```python
from build123d import *

# Parameters (mm, degrees)
SKETCH1_W           = 100
SKETCH1_H           = 20
BOSS_EXTRUDE1_DEPTH = 3
FILLET1_R           = 0.5
SKETCH2_R           = 1.5
CUT_EXTRUDE1_DEPTH  = 4


with BuildPart() as part:
    # Sketch1 → Boss-Extrude1 (new body)
    with BuildSketch(Plane(origin=(0, 0, 0), x_dir=(1, 0, 0), z_dir=(0, 1, 0))):
        Rectangle(SKETCH1_W, SKETCH1_H)
    extrude(amount=BOSS_EXTRUDE1_DEPTH)

    # Fillet1
    fillet1_edges = [part.edges().sort_by_distance(p)[0] for p in [
        (50, 3, 0),
        (0, 3, -10),
        (-50, 3, 0),
        (0, 0, -10),
        (50, 0, 0),
        (0, 0, 10),
        (-50, 0, 0),
        (0, 3, 10),
        (-50, 1.5, -10),
        (50, 1.5, -10),
        (50, 1.5, 10),
        (-50, 1.5, 10),
    ]]
    fillet(fillet1_edges, radius=FILLET1_R)

    # Sketch2 → Cut-Extrude1 (cut, through all)
    with BuildSketch(Plane.XZ):
        with Locations((45, 5)):
            Circle(SKETCH2_R)
    cut_extrude1 = extrude(amount=-CUT_EXTRUDE1_DEPTH, mode=Mode.SUBTRACT)

    # Mirror1: Cut-Extrude1 across plane
    add(cut_extrude1.mirror(Plane(origin=(0, 0, 0), x_dir=(0, 0, 1), z_dir=(1, 0, 0))), mode=Mode.SUBTRACT)


solid = part.part
```
Design review of the part built by this model. Coordinates are the model's own, in mm. Coordinates: 2 decimals unless noted, no trailing zeros. Order: outer loops, then holes, each group sorted by start corner. A loop starts at its lowest first (then second) coordinate and runs counter-clockwise, first axis right, second up. Notation, with made-up numbers: M 68.25,33 L 104.25,33 A13 cw 104.25,53 Z; hole C 66.5,63 d11. An arc over 180 degrees is marked long. Answer as a JSON object with one key per item and string values. Group by question number.
1) Add section B-B, the plane x = 45. Write out the cut boundary in (y, z), then the cut area to 3 significant figures.
2) Mouldability with a two-part tool opening along X and no side actions: class faces 1 (the cylindrical face through (43.5, 1.48, 5.07)), 2 (the flat face through (-50, 1, 0)), 3 (the flat face through (-1, 1, 10)) as pulls with the +X half, pulls with the -X half, needs draft (parallel to the pull), parting line crosses it, or undercut.
3) Add section A-A, the plane z = 5. Write out the cut boundary in (x, y), then the cut area to 3 significant figures.
4) Wall thickness on L1, parallel to Z at x = 45, y = 1.9; L2, parallel to X at y = 2.6, z = -3.25; L3, parallel to X at y = 0.2, z = 1.5: over which ranges is each line inside the solid? List them lowest first.
Computed values:
{
 "1": {"outline": "M 0,-9.5 A0.5 ccw 0.5,-10 L 2.5,-10 A0.5 ccw 3,-9.5 L 3,3.5 L 0,3.5 Z; M 0,6.5 L 3,6.5 L 3,9.5 A0.5 ccw 2.5,10 L 0.5,10 A0.5 ccw 0,9.5 Z", "area": "50.8 mm^2"},
 "2": {"face 1": "undercut", "face 2": "pulls with the -X half", "face 3": "needs draft"},
 "3": {"outline": "M -50,0.5 A0.5 ccw -49.5,0 L -46.5,0 L -46.5,3 L -49.5,3 A0.5 ccw -50,2.5 Z; M -43.5,0 L 43.5,0 L 43.5,3 L -43.5,3 Z; M 46.5,0 L 49.5,0 A0.5 ccw 50,0.5 L 50,2.5 A0.5 ccw 49.5,3 L 46.5,3 Z", "area": "282 mm^2"},
 "4": {"L1": "z = -10 to 3.5, 6.5 to 10", "L2": "x = -49.99 to 49.99", "L3": "x = -49.9 to 49.9"}
}
